```python
from build123d import *

# Parameters (mm, degrees)
BOSS_EXTRUDE1_DEPTH      = 10
BOSS_EXTRUDE1_DEPTH_BACK = 900
SKETCH2_R                = 7.75
CUT_EXTRUDE2_DEPTH       = 1.5
FILLET1_R                = 2.3
FILLET2_R                = 0.8


with BuildPart() as part:
    # Sketch1 → Boss-Extrude1 (new, two sides: drawn at the far end of the back side and taken through both)
    with BuildSketch(Plane.XY.offset(-BOSS_EXTRUDE1_DEPTH_BACK)):
        Polygon((0, 0), (30, 0), (30, 1.5), (1.5, 1.5), (1.5, 38.5), (40, 38.5), (40, 40), (0, 40), align=None)
    extrude(amount=BOSS_EXTRUDE1_DEPTH + BOSS_EXTRUDE1_DEPTH_BACK)

    # Sketch2 → Cut-Extrude2 (cut)
    with BuildSketch(Plane.XZ):
        with Locations(Location((15, -25, 0), (0, 0, 270))):
            Circle(SKETCH2_R)
        with Locations(Location((15, -60, 0), (0, 0, 270))):
            Circle(SKETCH2_R)
        with Locations(Location((15, -95, 0), (0, 0, 270))):
            Circle(SKETCH2_R)
        with Locations(Location((15, -130, 0), (0, 0, 270))):
            Circle(SKETCH2_R)
        with Locations(Location((15, -165, 0), (0, 0, 270))):
            Circle(SKETCH2_R)
        with Locations(Location((15, -200, 0), (0, 0, 270))):
            Circle(SKETCH2_R)
        with Locations(Location((15, -235, 0), (0, 0, 270))):
            Circle(SKETCH2_R)
        with Locations(Location((15, -270, 0), (0, 0, 270))):
            Circle(SKETCH2_R)
        with Locations(Location((15, -305, 0), (0, 0, 270))):
            Circle(SKETCH2_R)
        with Locations(Location((15, -340, 0), (0, 0, 270))):
            Circle(SKETCH2_R)
        with Locations(Location((15, -375, 0), (0, 0, 270))):
            Circle(SKETCH2_R)
        with Locations(Location((15, -410, 0), (0, 0, 270))):
            Circle(SKETCH2_R)
        with Locations(Location((15, -445, 0), (0, 0, 270))):
            Circle(SKETCH2_R)
        with Locations(Location((15, -480, 0), (0, 0, 270))):
            Circle(SKETCH2_R)
        with Locations(Location((15, -515, 0), (0, 0, 270))):
            Circle(SKETCH2_R)
        with Locations(Location((15, -550, 0), (0, 0, 270))):
            Circle(SKETCH2_R)
        with Locations(Location((15, -585, 0), (0, 0, 270))):
            Circle(SKETCH2_R)
        with Locations(Location((15, -620, 0), (0, 0, 270))):
            Circle(SKETCH2_R)
        with Locations(Location((15, -655, 0), (0, 0, 270))):
            Circle(SKETCH2_R)
        with Locations(Location((15, -690, 0), (0, 0, 270))):
            Circle(SKETCH2_R)
        with Locations(Location((15, -725, 0), (0, 0, 270))):
            Circle(SKETCH2_R)
        with Locations(Location((15, -760, 0), (0, 0, 270))):
            Circle(SKETCH2_R)
        with Locations(Location((15, -795, 0), (0, 0, 270))):
            Circle(SKETCH2_R)
        with Locations(Location((15, -830, 0), (0, 0, 270))):
            Circle(SKETCH2_R)
        with Locations(Location((15, -865, 0), (0, 0, 270))):
            Circle(SKETCH2_R)
    extrude(amount=-CUT_EXTRUDE2_DEPTH, mode=Mode.SUBTRACT)

    # Fillet1
    fillet1_edges = [part.edges().sort_by_distance(p)[0] for p in [
        (0, 40, -445),
        (0, 0, -445),
    ]]
    fillet(fillet1_edges, radius=FILLET1_R)

    # Fillet2
    fillet2_edges = [part.edges().sort_by_distance(p)[0] for p in [
        (1.5, 38.5, -445),
        (1.5, 1.5, -445),
    ]]
    fillet(fillet2_edges, radius=FILLET2_R)


solid = part.part
```
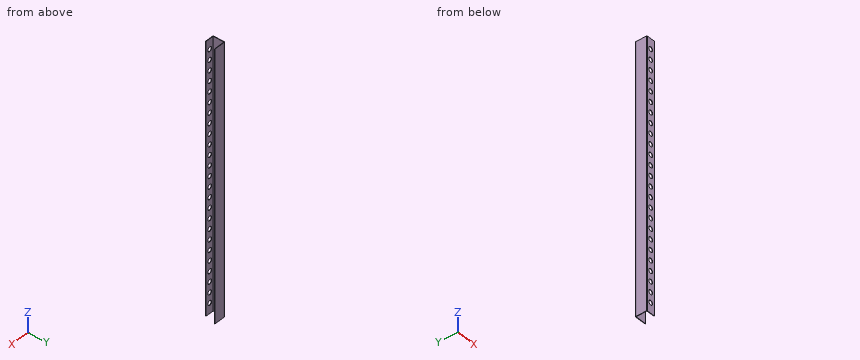
CAD build for the part. Positions are in the model's coordinates, mm. Coordinates: 2 decimals unless noted, no trailing zeros. Write each loop counter-clockwise with the first axis right and the second up, starting at its lowest first coordinate (ties: lowest second). Pieces come first, ordered by that corner, then holes. Notation, with made-up numbers: (82, 51) -> (92, 51) arc R15 ccw to (92, 74) -> close; hole circle Ø2 at (-19, -28.5). An arc over 180 degrees is marked (long way). Return JSON: item names as keys, results as strings. Group by question number.
Q1. Flat gauge pin, fed straight in: pin 1 (14 mm diameter, centred on x = 15, z = -655, fed in from -Y). Where does the tip first touch, or does it go through?
Q2. Cut at B-B, the plane y = 20. Give the cut face in (x, z).
Q3. Drill centre lines: line 1 (Y direction, x = 29, z = -79); line 2 (Y direction, x = 37.5, z = -51); line 3 (X direction, y = 32, z = -386). Where is each one in solid material? Low to high.
Q4. Cut at A-A, the plane z = -620. Give the cut face in (x, y), then the cut area to 3 significant figures.
Returned:
{
 "1": {"pin 1": "stops at y = 38.5"},
 "2": {"outline": "(0, -900) -> (1.5, -900) -> (1.5, 10) -> (0, 10) -> close"},
 "3": {"line 1": "y = 0 to 1.5, 38.5 to 40", "line 2": "y = 38.5 to 40", "line 3": "x = 0 to 1.5"},
 "4": {"outline": "(0, 2.3) arc R2.3 ccw to (2.3, 0) -> (7.25, 0) -> (7.25, 1.5) -> (2.3, 1.5) arc R0.8 cw to (1.5, 2.3) -> (1.5, 37.7) arc R0.8 cw to (2.3, 38.5) -> (40, 38.5) -> (40, 40) -> (2.3, 40) arc R2.3 ccw to (0, 37.7) -> close; (22.75, 0) -> (30, 0) -> (30, 1.5) -> (22.75, 1.5) -> close", "area": "135 mm2"}
}
